The listing builds one solid part. Answer for the finished solid, in the listing's coordinates (mm). Face numbers are marked on the shaded views. A direction names the side the tool comes from. Round coordinates to 2 decimals unless told otherwise and drop trailing zeros. Loops run counter-clockwise (first coordinate to the right, second up) from the corner with the lowest first, then second, coordinate; pieces in that order, holes last. Notation, with made-up numbers: M 33,0 L 83,0 A11 cw 83,18 Z; hole C 21,-0.5 d7. An arc over 180 degrees is marked long. Put each result on its own line as item: value. Start each with the question number.
(1) Section B-B, the plane z = -1.5 is taken. Determine the outline of the cut face in (x, y).
(2) Straight lines are drawn through the part: line 1 (Y direction, x = 36, z = -10); line 2 (X direction, y = -26.5, z = -13); line 3 (Z direction, x = 42.5, y = -26). For each, find the intervals that lie inside material, in ascending order.
(3) Section C-C, the plane x = 6 is taken. Determine the outline of the cut face in (y, z).
(4) Section D-D, the plane y = -14 is taken. Determine the outline of the cut face in (x, z), then the cut area to 3 significant figures.
(5) Section A-A, the plane y = -27 is taken. Determine the outline of the cut face in (x, z).
(6) Flat-ended cylindrical pins translate along their axes: P1, Ø1.5, axis at y = -23, z = -10.5, coming from the -X side; P2, Ø12, axis at x = 13, z = -11, coming from the +Y side; P3, Ø1, axis at y = -21, z = -9.5, coming from the +X side; P4, Ø15, axis at x = 42, z = -7, coming from the -Y side. Find the tip coordinate at first contact, or state that the pin passes through.
(7) Which of the six approach directions +Z, -Z, +X, -X, +Y, -Y give full straight-line access (tool end or side, diameter ignored) to the marked faces 1, 2 and 3?
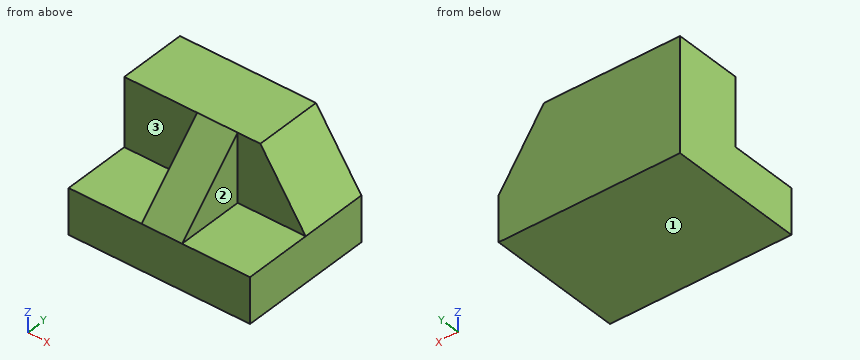
```python
from build123d import *

# Parameters (mm, degrees)
F0_W     = 50.8
F0_H     = 31.75
F1_DEPTH = 38.1
F2_W     = 19.05
F2_H     = 19.05
F3_DEPTH = 19.05
F4_W     = 20.428084
F4_H     = 19.05
F5_DEPTH = 19.05
F7_DEPTH = 25.4
F9_DEPTH = 25.4


with BuildPart() as f1:
    # F0 (on Front) → F1 (new body)
    with BuildSketch(Plane.XZ):
        with Locations((25.4, -15.875)):
            Rectangle(F0_W, F0_H)
    extrude(amount=F1_DEPTH)

    # F2 (on face) → F3 (cut)
    with BuildSketch(Plane.XY):
        with Locations((41.275, -28.575)):
            Rectangle(F2_W, F2_H)
    extrude(amount=-F3_DEPTH, mode=Mode.SUBTRACT)

    # F4 (on face) → F5 (cut)
    with BuildSketch(Plane.XY):
        with Locations((10.214042, -28.575)):
            Rectangle(F4_W, F4_H)
    extrude(amount=-F5_DEPTH, mode=Mode.SUBTRACT)

    # F6 (on face) → F7 (cut)
    with BuildSketch(Plane.YZ.offset(31.75)):
        Polygon((-38.1, -19.05), (-19.05, 0), (-38.1, 0), align=None)
    extrude(amount=-F7_DEPTH, mode=Mode.SUBTRACT)

    # F8 (on face) → F9 (cut)
    with BuildSketch(Plane.XZ.offset(19.05)):
        Polygon((50.8, 0), (38.1, 0), (50.8, -19.05), align=None)
    extrude(amount=-F9_DEPTH, mode=Mode.SUBTRACT)


solid = f1.part
```
Recorded:
1. outline: M 0,-19.05 L 20.43,-19.05 L 20.43,-20.55 L 31.75,-20.55 L 31.75,-19.05 L 39.1,-19.05 L 39.1,0 L 0,0 Z
2. line 1: y = -19.05 to 0
2. line 2: x = 20.43 to 31.75
2. line 3: z = -31.75 to -19.05
3. outline: M -38.1,-31.75 L 0,-31.75 L 0,0 L -19.05,0 L -19.05,-19.05 L -38.1,-19.05 Z
4. outline: M 0,-31.75 L 50.8,-31.75 L 50.8,-19.05 L 38.1,0 L 0,0 Z
4. area: 1,490 mm²
5. outline: M 0,-31.75 L 50.8,-31.75 L 50.8,-19.05 L 31.75,-19.05 L 31.75,-7.95 L 20.43,-7.95 L 20.43,-19.05 L 0,-19.05 Z
6. P1: stops at x = 20.43
6. P2: stops at y = 0
6. P3: stops at x = 31.75
6. P4: stops at y = -19.05
7. face 1: -Z, +X, -X, +Y, -Y
7. face 2: +Z, +X, -Y
7. face 3: +Z, -X, -Y
